Could you check a few things on this drawing? It's one solid part, dimensions in mm from its lowest x, y, z. Give positions to 0.01 mm unless a question says otherwise; leave off trailing zeros. Loops run counter-clockwise (first coordinate to the right, second up) from the corner with the lowest first, then second, coordinate; pieces in that order, holes last.
1. Thinking about a two-plate mould opening in X: for the marked faces 1, 2 and 3, which applies, +X half, -X half, draft (parallel to the pull), parting line (faces both ways), or undercut?
2. For P1, Ø4, axis at x = 4.5, y = 13.5, coming from the -Z side, with a flat end and sliding along its axis, tell me the tip position at first contact or that it passes through.
3. Imagine slicing it at A-A (x = 13.5). List the corners of the cut face in (y, z) for me, plus the area to 3 significant figures.
4. Imagine slicing it at D-D (y = 21.5). List the corners of the cut face in (x, z) for me, plus the area to 3 significant figures.
5. I need wall thicknesses on line 1 along Y through (x, z) = (13.5, 0.95); line 2 along Y through (x, z) = (14.5, 2.35). Which ranges of each line are inside material? Lowest first, please.
6. Imagine slicing it at C-C (z = 1.2). List the corners of the cut face in (x, y) for me.
7. Imagine slicing it at B-B (y = 4.5). List the corners of the cut face in (x, z) for me.
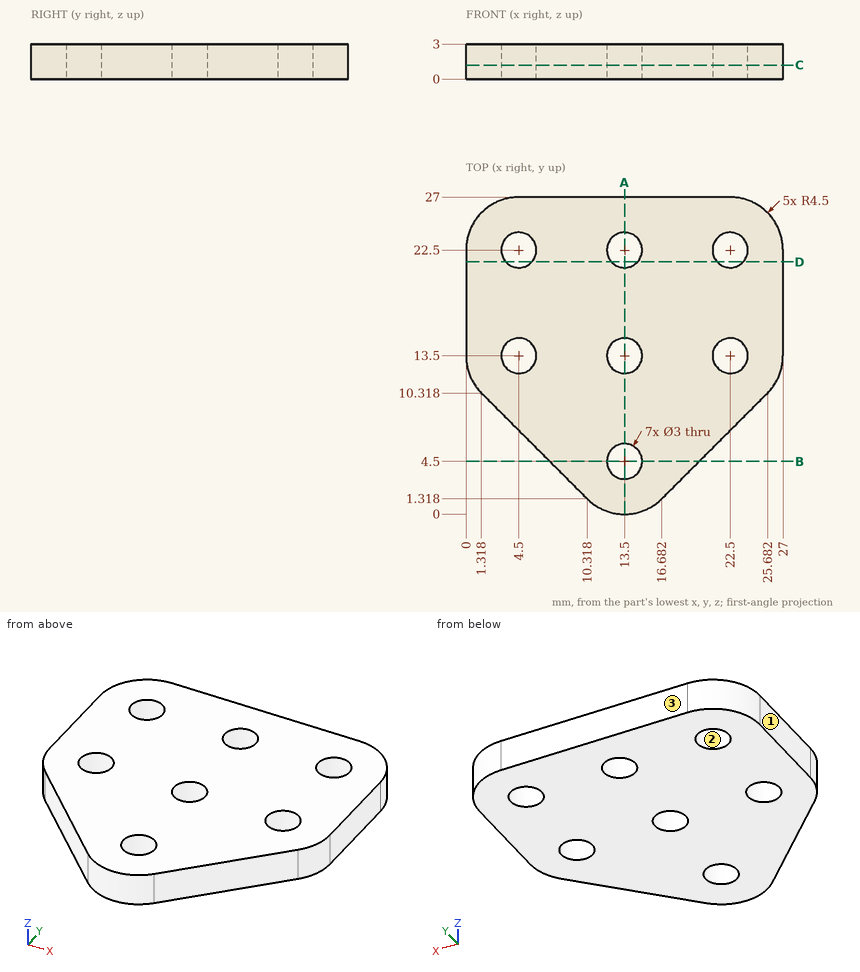
Derived:
1. face 1: -X half
1. face 2: undercut
1. face 3: draft
2. P1: stops at z = 0
3. outline: (0, 0) - (3, 0) - (3, 3) - (0, 3) - close; (6, 0) - (12, 0) - (12, 3) - (6, 3) - close; (15, 0) - (21, 0) - (21, 3) - (15, 3) - close; (24, 0) - (27, 0) - (27, 3) - (24, 3) - close
3. area: 54.0 mm2
4. outline: (0, 0) - (3.38, 0) - (3.38, 3) - (0, 3) - close; (5.62, 0) - (12.38, 0) - (12.38, 3) - (5.62, 3) - close; (14.62, 0) - (21.38, 0) - (21.38, 3) - (14.62, 3) - close; (23.62, 0) - (27, 0) - (27, 3) - (23.62, 3) - close
4. area: 60.9 mm2
5. line 1: y = 0 to 3, 6 to 12, 15 to 21, 24 to 27
5. line 2: y = 0.11 to 3.38, 5.62 to 12.38, 14.62 to 21.38, 23.62 to 27
6. outline: (0, 13.5) arc R4.5 ccw to (1.32, 10.32) - (10.32, 1.32) arc R4.5 ccw to (16.68, 1.32) - (25.68, 10.32) arc R4.5 ccw to (27, 13.5) - (27, 22.5) arc R4.5 ccw to (22.5, 27) - (4.5, 27) arc R4.5 ccw to (0, 22.5) - close; hole circle Ø3 at (4.5, 13.5); hole circle Ø3 at (4.5, 22.5); hole circle Ø3 at (13.5, 4.5); hole circle Ø3 at (13.5, 13.5); hole circle Ø3 at (13.5, 22.5); hole circle Ø3 at (22.5, 13.5); hole circle Ø3 at (22.5, 22.5)
7. outline: (7.14, 0) - (12, 0) - (12, 3) - (7.14, 3) - close; (15, 0) - (19.86, 0) - (19.86, 3) - (15, 3) - close
